Could you check a few things on this model? Use its own coordinates, in mm. Face numbers are marked on the shaded views. A direction names the side the tool comes from. Give positions to 0.01 mm unless a question says otherwise; leave off trailing zeros. Write each loop counter-clockwise with the first axis right and the second up, starting at its lowest first coordinate (ties: lowest second). Pieces come first, ordered by that corner, then holes. Notation, with made-up numbers: M 56,45.25 L 75,45.25 A28 cw 75,67.25 Z; hole C -33.75,25 d3. An arc over 180 degrees is marked long. One line per item, written item: value.
```python
from build123d import *

# Parameters (mm, degrees)
SKETCH_4_R          = 2
CUT_EXTRUDE_1_DEPTH = 20


with BuildPart() as part:
    # Эскиз1 → Повернуть11 (revolve)
    with BuildSketch(Plane.XY):
        Polygon((-30, -10), (0, -10), (0, 0), (-20.4, 0), (-22, -1.6), (-22, -5), (-30, -5), align=None)
    revolve(axis=Axis((0, 0, 0), (0, -1, 0)))

    # Эскиз4 → Вырез-Вытянуть1 (cut)
    with BuildSketch(Plane(origin=(0, -5, 0), x_dir=(1, 0, 0), z_dir=(0, 1, 0))):
        with Locations(Location((0, 26, 0), (0, 0, 180))):
            Circle(SKETCH_4_R)
        with Locations(Location((18.384776311, 18.384776311, 0), (0, 0, 180))):
            Circle(SKETCH_4_R)
        with Locations(Location((26, 0, 0), (0, 0, 180))):
            Circle(SKETCH_4_R)
        with Locations(Location((18.384776311, -18.384776311, 0), (0, 0, 180))):
            Circle(SKETCH_4_R)
        with Locations(Location((0, -26, 0), (0, 0, 180))):
            Circle(SKETCH_4_R)
        with Locations(Location((-18.384776311, -18.384776311, 0), (0, 0, 180))):
            Circle(SKETCH_4_R)
        with Locations(Location((-26, 0, 0), (0, 0, 180))):
            Circle(SKETCH_4_R)
        with Locations(Location((-18.384776311, 18.384776311, 0), (0, 0, 180))):
            Circle(SKETCH_4_R)
    extrude(amount=-CUT_EXTRUDE_1_DEPTH, mode=Mode.SUBTRACT)


solid = part.part
```
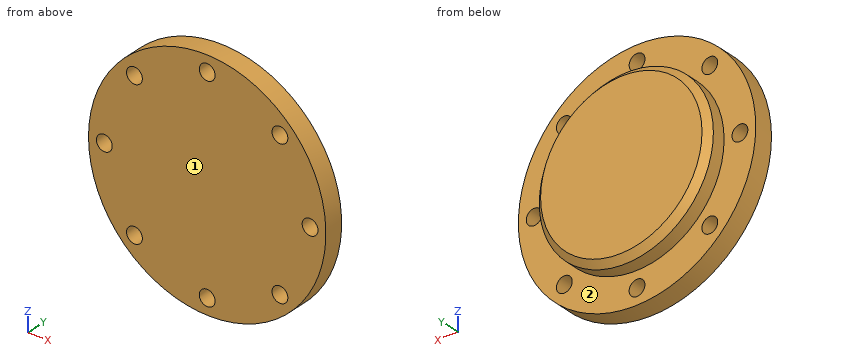
1) If we section it at C-C, the plane z = -26: Write out the boundary of the cut face in (x, y).
Outcome:
outline: M -14.97,-10 L -2,-10 L -2,-5 L -14.97,-5 Z; M 2,-10 L 14.97,-10 L 14.97,-5 L 2,-5 Z
2) If we section it at D-D, the plane x = -26: Write out the boundary of the cut face in (y, z), then the cut area to 3 significant figures.
Outcome:
outline: M -10,-14.97 L -5,-14.97 L -5,-2 L -10,-2 Z; M -10,2 L -5,2 L -5,14.97 L -10,14.97 Z
area: 130 mm^2
3) If we section it at A-A, the plane x = 0: Write out the boundary of the cut face in (y, z), then the cut area to 3 significant figures.
Outcome:
outline: M -10,-30 L -5,-30 L -5,-28 L -10,-28 Z; M -10,-24 L -5,-24 L -5,-22 L -1.6,-22 L 0,-20.4 L 0,20.4 L -1.6,22 L -5,22 L -5,24 L -10,24 Z; M -10,28 L -5,28 L -5,30 L -10,30 Z
area: 477 mm^2
4) I'm going to push flat-ended pins straight in: pin 1 (6.5 mm diameter, centred on x = -18.38, z = 18.38, fed in from +Y); pin 2 (2 mm diameter, centred on x = 22.5, y = -4.5, fed in from +Z); pin 3 (3 mm diameter, centred on x = -13.5, y = -6.5, fed in from -Z); pin 4 (3 mm diameter, centred on x = 26, z = 0, fed in from -Y). Where does each tip first touch, or does it pass through?
Outcome:
pin 1: stops at y = -5
pin 2: stops at z = 20.78
pin 3: stops at z = -27.5
pin 4: passes through
5) On a 3-axis mill with a long thin cutter (end or side, diameter ignored), from which of +Z, -Z, +X, -X, +Y, -Y can I reach the whole of each face in a straight line? I mean the marked faces 1 and 2. Say none if no direction works.
Outcome:
face 1: +Z, -Z, +X, -X, -Y
face 2: +Y
6) Please list where these lines run through material, in increasing order: L1, parallel to Z at x = 0, y = -6.35; L2, parallel to X at y = -5.25, z = -18.5; L3, parallel to Y at x = 8.5, z = 24. Write a range as from..to.
Outcome:
L1: z = -30..-28, -24..24, 28..30
L2: x = -23.62..-20.38, -16.39..16.39, 20.38..23.62
L3: y = -10..-5
7) If we section it at B-B, the plane z = 0: Write out the boundary of the cut face in (x, y), then the cut area to 3 significant figures.
Outcome:
outline: M -30,-10 L -28,-10 L -28,-5 L -30,-5 Z; M -24,-10 L 24,-10 L 24,-5 L 22,-5 L 22,-1.6 L 20.4,0 L -20.4,0 L -22,-1.6 L -22,-5 L -24,-5 Z; M 28,-10 L 30,-10 L 30,-5 L 28,-5 Z
area: 477 mm^2
